Design review of the part built by this model. Coordinates are the model's own, in mm. A direction names the side the tool comes from. Coordinates: 2 decimals unless noted, no trailing zeros. Write each loop counter-clockwise with the first axis right and the second up, starting at its lowest first coordinate (ties: lowest second). Pieces come first, ordered by that corner, then holes.
Q1. Take a section at B-B (z = -12). Give the boundary of the cut face in (x, y), and give its area (3 significant figures).
Q2. Machinability: for faces 5 (the cylindrical face through (-0.759, 2.583, -1.972)), 6 (the flat face through (12.5, 8, -36)), 7 (the flat face through (39.87, 6, -7)), 8 (the flat face through (9.5, 8, -42)), 9 (the flat face through (2.4, 3.2, -4)), which of the approach directions +Z, -Z, +X, -X, +Y, -Y give a long, thin tool a straight path to every point of the face, cutting with its end or side? Answer none if there is none.
Q3. Take a section at A-A (x = 35.37). Give the boundary of the cut face in (y, z).
Q4. Take a section at D-D (y = 13.5). Give the boundary of the cut face in (x, z), and give its area (3 significant figures).
Q5. Insertion check: pin 1 (5 mm diameter, centred on x = 34.5, y = 8.5, fed in from -Z); pin 2 (4.5 mm diameter, centred on x = 0, z = -11.5, fed in from -Y); pin 3 (3 mm diameter, centred on x = 19.5, y = 6, fed in from -Z). Each pin has a flat end and moves straight along its axis. Give the tip position at first contact, or say it passes through.
Q6. For probe 1 along X at (y, z) = (4.5, -5); probe 2 along Z at (x, y) = (-4.5, 5); probe 3 along X at (y, z) = (13, -36), list the stretches that pass through material, from the lowest coordinate up.
Q7. Take a section at C-C (x = 0). Give the boundary of the cut face in (y, z), and give its area (3 significant figures).
Q8. Mouldability with a two-part tool opening along Z and no side actions: class faces 1 (the flat face through (5.53, 5.92, -29.72)), 2 (the flat face through (-9.5, 8, -42)), 3 (the flat face through (35, 12, -7)), 4 (the flat face through (0, 10, -52.75)) as pulls with the +Z half, pulls with the -Z half, needs draft (parallel to the pull), parting line crosses it, or undercut.
```python
from build123d import *

# Parameters (mm, degrees)
SKETCH_1_W          = 19
SKETCH_1_H          = 14
EXTRUDE_1_DEPTH     = 12
CUT_EXTRUDE_2_REACH = 72.284
SKETCH_4_R          = 1.5
SKETCH_5_W          = 19
SKETCH_5_H          = 14
EXTRUDE_2_DEPTH     = 5
CUT_EXTRUDE_4_REACH = 73.308
SKETCH_6_R          = 3
SKETCH_7_R          = 3.5
CUT_EXTRUDE_5_DEPTH = 4
CHAMFER_1_SIZE      = 4
CHAMFER_2_SIZE      = 8


with BuildPart() as part:
    # 草图1 → 凸台-拉伸1 (new body)
    with BuildSketch(Plane(origin=(0, 0, 0), x_dir=(1, 0, 0), z_dir=(0, 1, 0))):
        Polygon((-30.87, 10.5), (-12.5, 10.5), (-12.5, 52.75), (12.5, 52.75), (12.5, 10.5), (30.87, 10.5), (30.87, 4), (39.87, 4), (39.87, 10.5), (44.87, 10.5), (44.87, 0), (-44.87, 0), (-44.87, 10.5), (-39.87, 10.5), (-39.87, 4), (-30.87, 4), align=None)
        with Locations((0, 41.75)):
            Rectangle(SKETCH_1_W, SKETCH_1_H, mode=Mode.SUBTRACT)
        Polygon((-7.5, 31.75), (7.5, 31.75), (7.5, 7.5), (7.5, 4), (-7.5, 4), (-7.5, 7.5), align=None, mode=Mode.SUBTRACT)
    extrude(amount=EXTRUDE_1_DEPTH)

    # 草图4 → 切除-拉伸2 (cut, up to next)
    with BuildSketch(Plane.XY, mode=Mode.PRIVATE) as cut_extrude_2_sk1:
        with Locations((-35.37, 5)):
            Circle(SKETCH_4_R)
    cut_extrude_2_tool1 = extrude(cut_extrude_2_sk1.sketch, amount=-CUT_EXTRUDE_2_REACH, mode=Mode.PRIVATE) & part.part
    # 草图4 → 切除-拉伸2 (cut, up to next)
    with BuildSketch(Plane.XY, mode=Mode.PRIVATE) as cut_extrude_2_sk2:
        with Locations((35.37, 5)):
            Circle(SKETCH_4_R)
    cut_extrude_2_tool2 = extrude(cut_extrude_2_sk2.sketch, amount=-CUT_EXTRUDE_2_REACH, mode=Mode.PRIVATE) & part.part
    add(cut_extrude_2_tool1.solids().sort_by_distance((-35.37, 5, 0))[0], mode=Mode.SUBTRACT)
    add(cut_extrude_2_tool2.solids().sort_by_distance((35.37, 5, 0))[0], mode=Mode.SUBTRACT)

    # 草图5 → 凸台-拉伸2 (add)
    with BuildSketch(Plane(origin=(0, 12, 0), x_dir=(1, 0, 0), z_dir=(0, 1, 0))):
        Polygon((-39.87, 10.5), (-30.87, 10.5), (-12.5, 10.5), (-12.5, 52.75), (12.5, 52.75), (12.5, 10.5), (30.87, 10.5), (39.87, 10.5), (44.87, 10.5), (44.87, 0), (-44.87, 0), (-44.87, 10.5), align=None)
        with Locations((0, 41.75)):
            Rectangle(SKETCH_5_W, SKETCH_5_H, mode=Mode.SUBTRACT)
    extrude(amount=EXTRUDE_2_DEPTH)

    # 切除-拉伸4: up to this face of the body (flat: up to its plane)
    cut_extrude_4_end = Plane(part.part.faces().sort_by_distance((0, 6, -31.75))[0])
    # 草图6 → 切除-拉伸4 (cut, up to the picked face)
    with BuildSketch(Plane(origin=(0, 0, -52.75), x_dir=(-1, 0, 0), z_dir=(0, 0, -1)), mode=Mode.PRIVATE) as cut_extrude_4_sk1:
        with Locations((0, 6)):
            Circle(SKETCH_6_R)
    cut_extrude_4_tool1 = split(extrude(cut_extrude_4_sk1.sketch, amount=-CUT_EXTRUDE_4_REACH, mode=Mode.PRIVATE), bisect_by=cut_extrude_4_end, keep=Keep.BOTH, mode=Mode.PRIVATE)
    add(cut_extrude_4_tool1.solids().sort_by(Axis((0, 6, -52.75), (0, 0, 1)))[0], mode=Mode.SUBTRACT)

    # 草图7 → 切除-拉伸5 (cut)
    with BuildSketch(Plane.XY):
        with Locations((0, 6)):
            Circle(SKETCH_7_R)
    extrude(amount=-CUT_EXTRUDE_5_DEPTH, mode=Mode.SUBTRACT)

    # 倒角1
    chamfer_1_edges = [part.edges().sort_by_distance(p)[0] for p in [
        (-7.5, 6, -4),
        (7.5, 6, -4),
        (7.5, 6, -31.75),
        (-7.5, 6, -31.75),
    ]]
    chamfer(chamfer_1_edges, length=CHAMFER_1_SIZE - 0.0001)  # a hair under: the kernel refuses the full size

    # 倒角2
    chamfer_2_edges = [part.edges().sort_by_distance(p)[0] for p in [
        (-12.5, 8.5, -10.5),
        (12.5, 8.5, -10.5),
    ]]
    chamfer(chamfer_2_edges, length=CHAMFER_2_SIZE)


solid = part.part
```
Response:
1. outline: (-19, 0) - (-7.5, 0) - (-7.5, 12) - (7.5, 12) - (7.5, 0) - (19, 0) - (19, 17) - (-19, 17) - close
1. area: 466 mm2
2. face 5: +Z
2. face 6: -Z, +X, +Y, -Y
2. face 7: -Z, -Y
2. face 8: +Y, -Y
2. face 9: -Y
3. outline: (0, -4) - (3.5, -4) - (3.5, 0) - (0, 0) - close; (6.5, -4) - (12, -4) - (12, -10.5) - (17, -10.5) - (17, 0) - (6.5, 0) - close
4. outline: (-44.87, -10.5) - (-20.5, -10.5) - (-12.5, -18.5) - (-12.5, -52.75) - (12.5, -52.75) - (12.5, -18.5) - (20.5, -10.5) - (44.87, -10.5) - (44.87, 0) - (-44.87, 0) - close; hole (-9.5, -48.75) - (9.5, -48.75) - (9.5, -34.75) - (-9.5, -34.75) - close
4. area: 1,800 mm2
5. pin 1: stops at z = -4
5. pin 2: stops at y = 12
5. pin 3: stops at z = -13
6. probe 1: x = -44.87 to -39.87, -30.87 to -4.5, 4.5 to 30.87, 39.87 to 44.87
6. probe 2: z = -52.75 to -48.75, -34.75 to -30.75, -5 to 0
6. probe 3: x = -12.5 to -9.5, 9.5 to 12.5
7. outline: (0, -52.75) - (3, -52.75) - (3, -48.75) - (0, -48.75) - close; (0, -34.75) - (3, -34.75) - (3, -31.75) - (0, -31.75) - close; (0, -4) - (2.5, -4) - (2.5, 0) - (0, 0) - close; (9, -52.75) - (17, -52.75) - (17, -48.75) - (9, -48.75) - close; (9, -34.75) - (17, -34.75) - (17, 0) - (9.5, 0) - (9.5, -4) - (12, -4) - (12, -31.75) - (9, -31.75) - close
7. area: 256 mm2
8. face 1: undercut
8. face 2: undercut
8. face 3: needs draft
8. face 4: pulls with the -Z half
